from build123d import *

# Parameters (mm, degrees)
SKETCH1_W           = 1219.2
SKETCH1_H           = 635
BOSS_EXTRUDE1_DEPTH = 152.4
LPATTERN3_COUNT     = 3
LPATTERN3_PITCH     = 609.6
LPATTERN3_2_COUNT   = 2
LPATTERN3_2_PITCH   = 635


with BuildPart() as part:
    # Sketch1 → Boss-Extrude1 (new body)
    with BuildSketch(Plane(origin=(0, 0, 0), x_dir=(1, 0, 0), z_dir=(0, 1, 0))):
        Rectangle(SKETCH1_W, SKETCH1_H)
    extrude(amount=BOSS_EXTRUDE1_DEPTH)


with BuildPart() as body_2:
    # Sketch3 → Revolve1 (revolve)
    with BuildSketch(Plane(origin=(0, -50.8, 0), x_dir=(-1, 0, 0), z_dir=(0, -1, 0))):
        with BuildLine():
            Line((-736.6, 317.5), (-482.6, 317.5))
            ThreePointArc((-482.6, 317.5), (-609.6, 444.5), (-736.6, 317.5))
        make_face()
    revolve(axis=Axis((-609.6, -50.8, -317.5), (1, 0, 0)))


with BuildPart() as lpattern3_1:
    # LPattern3: pattern copy
    add(body_2.part.moved(Location(Vector(-1, 0, 0) * (1 * LPATTERN3_PITCH))))


with BuildPart() as lpattern3_2:
    # LPattern3: pattern copy
    add(body_2.part.moved(Location(Vector(-1, 0, 0) * (2 * LPATTERN3_PITCH))))


with BuildPart() as lpattern3_2_1:
    # LPattern3 2: pattern copy
    add(body_2.part.moved(Location(Vector(0, 0, 1) * (1 * LPATTERN3_2_PITCH))))


with BuildPart() as lpattern3_2_2:
    # LPattern3 2: pattern copy
    add(lpattern3_1.part.moved(Location(Vector(0, 0, 1) * (1 * LPATTERN3_2_PITCH))))


with BuildPart() as lpattern3_2_3:
    # LPattern3 2: pattern copy
    add(lpattern3_2.part.moved(Location(Vector(0, 0, 1) * (1 * LPATTERN3_2_PITCH))))


with BuildPart() as part_1:
    add(part.part)

    # Intersect1: read off the stored shape, not the designer's step
    # Intersect1: cut body 2, LPattern3_1, LPattern3_2, LPattern3 2_1, LPattern3 2_2, LPattern3 2_3
    add(body_2.part, mode=Mode.SUBTRACT)
    add(lpattern3_1.part, mode=Mode.SUBTRACT)
    add(lpattern3_2.part, mode=Mode.SUBTRACT)
    add(lpattern3_2_1.part, mode=Mode.SUBTRACT)
    add(lpattern3_2_2.part, mode=Mode.SUBTRACT)
    add(lpattern3_2_3.part, mode=Mode.SUBTRACT)


solid = part_1.part
Read the model definition and answer for the solid it produces. Units are mm, in the model's axes. Coordinates: 2 decimals unless noted, no trailing zeros. Order: outer loops, then holes, each group sorted by start corner. A loop starts at its lowest first (then second) coordinate and runs counter-clockwise, first axis right, second up. Notation, with made-up numbers: (-35, 54) -> (13, 54) arc R10 ccw to (13, 71) -> close; hole circle Ø8 at (88, -23.5). An arc over 180 degrees is marked (long way). Answer as a JSON object with one key per item and string values.
1) Consider line 1 along X through (y, z) = (36.5, -273); line 2 along Z through (x, y) = (-82, 14). Determine where each line is inside the solid, lowest interval first. Write a range as from..to.
Model answer:
{"line 1": "x = -528.81..-80.79, 80.79..528.81", "line 2": "z = -245.35..245.35"}
2) A cutting plane is placed at D-D, the plane x = 508. Determine the outline of the cut face in (y, z).
Model answer:
{"outline": "(0, -260.7) arc R76.2 cw to (25.4, -317.5) -> (152.4, -317.5) -> (152.4, 317.5) -> (25.4, 317.5) arc R76.2 cw to (0, 260.7) -> close"}
3) A cutting plane is placed at C-C, the plane z = 241. Determine the outline of the cut face in (x, y), plus the area to 3 significant figures.
Model answer:
{"outline": "(-609.6, 50.57) arc R101.37 cw to (-521.87, 0) -> (-87.73, 0) arc R101.37 cw to (87.73, 0) -> (521.87, 0) arc R101.37 cw to (609.6, 50.57) -> (609.6, 152.4) -> (-609.6, 152.4) -> close", "area": "173,000 mm²"}
4) A cutting plane is placed at B-B, the plane x = -517. Determine the outline of the cut face in (y, z), plus the area to 3 significant figures.
Model answer:
{"outline": "(0, -246.98) arc R86.92 cw to (36.12, -317.5) -> (152.4, -317.5) -> (152.4, 317.5) -> (36.12, 317.5) arc R86.92 cw to (0, 246.98) -> close", "area": "93,200 mm²"}
5) A cutting plane is placed at A-A, the plane y = 36. Determine the outline of the cut face in (x, z).
Model answer:
{"outline": "(-609.6, -224.79) arc R92.71 cw to (-516.89, -317.5) -> (-92.71, -317.5) arc R92.71 cw to (92.71, -317.5) -> (516.89, -317.5) arc R92.71 cw to (609.6, -224.79) -> (609.6, 224.79) arc R92.71 cw to (516.89, 317.5) -> (92.71, 317.5) arc R92.71 cw to (-92.71, 317.5) -> (-516.89, 317.5) arc R92.71 cw to (-609.6, 224.79) -> close"}
